The listing builds one solid part. Answer for the finished solid, in the listing's coordinates (mm). A direction names the side the tool comes from. Give positions to 0.01 mm unless a question says otherwise; leave off trailing zeros. Loops run counter-clockwise (first coordinate to the right, second up) from the corner with the lowest first, then second, coordinate; pieces in that order, holes last. Notation, with made-up numbers: M 52,-27.75 L 74,-27.75 A10 ccw 74,-22.75 Z; hole C 41,-19.75 d11. An arc over 180 degrees is marked long. One line per item, written item: value. Start each with the question number.
Q1. A cutting plane is placed at B-B, the plane y = 13.75. Determine the outline of the cut face in (x, z).
Q2. A cutting plane is placed at A-A, the plane z = -6.5. Determine the outline of the cut face in (x, y).
Q3. Flat-ended cylindrical pins translate along their axes: pin 1 (6 mm diameter, centred on y = 11.5, z = -7, fed in from -X); pin 2 (3 mm diameter, centred on x = 17.5, z = -13, fed in from -Y); pin 3 (1 mm diameter, centred on y = 6, z = -6, fed in from +X). Find the tip coordinate at first contact, or state that the pin passes through.
Q4. The mould has two halves that part along X. Classify faces 4 (the flat face through (16.67, -0.76, -7.95)), 5 (the flat face through (19, 0, -6)), 6 (the cylindrical face through (21.2, 11.83, -8.92)): +X half, -X half, draft (parallel to the pull), parting line (faces both ways), or undercut.
Q5. For faces 1 (the flat face through (17.472, -0.76, -6.187)), 2 (the cylindrical face through (19.396, -0.76, -8.051)), 3 (the flat face through (14, 12, -14)), determine the directions among +Z, -Z, +X, -X, +Y, -Y from which every point of the face is accessible in a straight line to the end or side of a thin tool.
Q6. A cutting plane is placed at D-D, the plane z = -12. Determine the outline of the cut face in (x, y).
Q7. Consider L1, parallel to Y at x = 21.5, z = -6; L2, parallel to Z at x = 12.25, y = 4.75; L3, parallel to Z at x = 18.5, y = 8. Determine where each line is inside the solid, lowest interval first.
Q8. A cutting plane is placed at C-C, the plane x = 18.25. Determine the outline of the cut face in (y, z).
from build123d import *

# Parameters (mm, degrees)
BOSS_EXTRUDE1_DEPTH = 24
BOSS_EXTRUDE2_START = 1.5
BOSS_EXTRUDE2_DEPTH = 1.5


with BuildPart() as part:
    # Sketch1 → Boss-Extrude1 (new body)
    with BuildSketch(Plane(origin=(0, 0, 0), x_dir=(1, 0, 0), z_dir=(0, 1, 0))):
        with BuildLine():
            Line((11.313708499, 11.313708499), (16.263455967, 16.263455967))
            ThreePointArc((16.263455967, 16.263455967), (21.249229248, 8.801718944), (23, 0))
            Line((23, 0), (16, 0))
            ThreePointArc((16, 0), (14.78207252, 6.122934918), (11.313708499, 11.313708499))
        make_face()
    extrude(amount=BOSS_EXTRUDE1_DEPTH)

    # Sketch4 → Boss-Extrude2 (add)
    with BuildSketch(Plane.XZ.offset(BOSS_EXTRUDE2_START)):
        with BuildLine():
            Line((14.44136455, -6.888177549), (18.954290971, -9.040733033))
            ThreePointArc((18.954290971, -9.040733033), (19.401470183, -8.03635208), (19.795471313, -7.009944044))
            Line((19.795471313, -7.009944044), (15.082263857, -5.340909748))
            ThreePointArc((15.082263857, -5.340909748), (14.78207252, -6.122934918), (14.44136455, -6.888177549))
        make_face()
    extrude(amount=-BOSS_EXTRUDE2_DEPTH)


solid = part.part
Answer block:
1. outline: M 11.31,-11.31 L 16.26,-16.26 A23 ccw 23,0 L 16,0 A16 cw Z
2. outline: M 14.62,-1.5 L 18.36,-1.5 L 18.36,0 L 22.06,0 L 22.06,24 L 14.62,24 Z
3. pin 1: x = 12.49
3. pin 2: y = 0
3. pin 3: x = 22.33
4. face 4: -X half
4. face 5: draft
4. face 6: +X half
5. face 1: +Z, +X, -Y
5. face 2: -Z, +X, -Y
5. face 3: -Z, -X, +Y, -Y
6. outline: M 12,0 L 19.62,0 L 19.62,24 L 12,24 Z
7. L1: 0 to 24
7. L2: -12.25 to -10.29
7. L3: -13.67 to 0
8. outline: M -1.5,-8.7 L 0,-8.7 L 0,-14 L 24,-14 L 24,0 L 0,0 L 0,-6.46 L -1.5,-6.46 Z
